Input: part model. Units: mm. Frame: model coordinates. A direction names the side the tool comes from. Coordinates: 2 decimals unless noted, no trailing zeros. Loops run counter-clockwise (first coordinate to the right, second up) from the corner with the lowest first, then second, coordinate; pieces in that order, holes last. Notation, with made-up numbers: (5, 8) - (39, 8) arc R13 ccw to (39, 31) - close; hole circle Ø3 at (-16.5, 26). An arc over 180 degrees is marked (long way). Answer as CSV lines item,"result". Start each with the question number.
```python
from build123d import *

# Parameters (mm, degrees)
F1_DEPTH  = 3.5
F2_W      = 29
F2_H      = 9
F3_DEPTH  = 4
F4_W      = 29
F4_H      = 9
F5_DEPTH  = 4
F6_SIZE   = 2
F7_W      = 4
F7_H      = 15
F8_DEPTH  = 3
F9_SIZE   = 2
F11_DEPTH = 29
F12_R     = 3


with BuildPart() as f1:
    # F0 (on Top) → F1 (new body)
    with BuildSketch(Plane.XY):
        Polygon((-4.25, 12.1511180716), (-18, 12.1511180716), (-18, -16.8488819284), (-11.125, -16.8488819284), (-11.125, -12.8488819284), (11.125, -12.8488819284), (11.125, -16.8488819284), (18, -16.8488819284), (18, 12.1511180716), (4.25, 12.1511180716), (4.25, 7.1511180716), (-4.25, 7.1511180716), align=None)
    extrude(amount=F1_DEPTH)

    # F2 (on face) → F3 (join)
    with BuildSketch(Plane(origin=(-18, 0, 0), x_dir=(0, -1, 0), z_dir=(-1, 0, 0))):
        with Locations((2.3488819284, -1)):
            Rectangle(F2_W, F2_H)
    extrude(amount=F3_DEPTH)

    # F4 (on face) → F5 (join)
    with BuildSketch(Plane.YZ.offset(18)):
        with Locations((-2.3488819284, -1)):
            Rectangle(F4_W, F4_H)
    extrude(amount=F5_DEPTH)

    # F6
    f6_edges = [f1.edges().sort_by_distance(p)[0] for p in [
        (-14.5625, -16.848882, 0),
        (14.5625, -16.848882, 0),
    ]]
    chamfer(f6_edges, length=F6_SIZE)

    # F7 (on face) → F8 (join)
    with BuildSketch(Plane(origin=(0, 0, -5.5), x_dir=(1, 0, 0), z_dir=(0, 0, -1))):
        with Locations((20, 2.3488819284)):
            Rectangle(F7_W, F7_H)
        with Locations((-20, 2.3488819284)):
            Rectangle(F7_W, F7_H)
    extrude(amount=F8_DEPTH)

    # F9
    f9_edges = [f1.edges().sort_by_distance(p)[0] for p in [
        (18, -16.848882, -1.75),
        (-18, -16.848882, -1.75),
    ]]
    chamfer(f9_edges, length=F9_SIZE)

    # F10 (on face) → F11 (join, through all)
    with BuildSketch(Plane(origin=(0, 12.1511180716, 0), x_dir=(-1, 0, 0), z_dir=(0, 1, 0))):
        Polygon((25, -5.5), (22, 3.5), (22, -5.5), align=None)
        Polygon((-22, -5.5), (-22, 3.5), (-25, -5.5), align=None)
    extrude(amount=-F11_DEPTH)

    # F12
    f12_edges = [f1.edges().sort_by_distance(p)[0] for p in [
        (-22, -2.348882, 3.5),
        (22, -2.348882, 3.5),
    ]]
    fillet(f12_edges, radius=F12_R)


solid = f1.part
```
Item 1: Section query D-D, the plane x = 16. Output: boundary loops of the cut face in (y, z), and give its area (3 significant figures).
Item 2: Set-up query: faces 4 (the flat face through (-20, 5.151, -7)), 5 (the flat face through (-11.125, -14, 2)), 6 (the flat face through (-22, -2, -7)), 7 (the flat face through (20, -9.849, -7)), 8 (the flat face through (-18.986, -15.835, -2.636)). Return all of +Z, -Z, +X, -X, +Y, -Y with unobstructed straight access to the full face (end or side cutting, diameter ignored); none if empty.
Item 3: Contact query for flat-ended pins moving along their axis: P1, Ø0.9, axis at y = -6, z = -6.5, coming from the -X side; P2, Ø1.5, axis at y = -4, z = 1.5, coming from the +X side; P3, Ø2, axis at y = 5.5, z = -2, coming from the +X side; P4, Ø2.5, axis at y = -5, z = -6.5, coming from the +X side. Output: stop coordinate, or through.
Item 4: Section query A-A, the plane z = -1. Output: boundary loops of the cut face in (x, y).
Item 5: Section query C-C, the plane y = -12.25. Output: boundary loops of the cut face in (x, z).
Item 6: Section query B-B, the plane y = 8. Output: boundary loops of the cut face in (x, z).
Item 7: Draft query along X for faces 1 (the cylindrical face through (-21.61, -2.55, 2.92)), 2 (the flat face through (20, -2, -8.5)), 3 (the flat face through (0, -1, 0)). Return one class per face: pulls with the +X half, pulls with the -X half, needs draft (parallel to the pull), parting line crosses it, or undercut.
Item 8: Material intervals for probe 1 along Z at (x, y) = (15, -7); probe 2 along X at (y, z) = (-8.75, -5.75); probe 3 along X at (y, z) = (8.5, 1.5), sorted ascending.
Response values:
1,outline,"(-16.85, 2) - (-14.85, 0) - (12.15, 0) - (12.15, 3.5) - (-16.85, 3.5) - close"
1,area,"99.5 mm²"
2,face 4,"-Z, +X, -X, +Y"
2,face 5,"+Z, -Z, -Y"
2,face 6,"-Z, -X, +Y, -Y"
2,face 7,"-Z, +X, -X, -Y"
2,face 8,"-Z, -Y"
3,P1,"stops at x = -22"
3,P2,"stops at x = 22.92"
3,P3,"stops at x = 24.17"
3,P4,"stops at x = 25"
4,outline,"(-23.5, -16.85) - (-20, -16.85) - (-18, -14.85) - (-18, 12.15) - (-23.5, 12.15) - close; (18, -14.85) - (20, -16.85) - (23.5, -16.85) - (23.5, 12.15) - (18, 12.15) - close"
5,outline,"(-25, -5.5) - (-18, -5.5) - (-18, 0) - (18, 0) - (18, -5.5) - (25, -5.5) - (22.68, 1.45) arc R3 ccw to (19.84, 3.5) - (-19.84, 3.5) arc R3 ccw to (-22.68, 1.45) - close"
6,outline,"(-25, -5.5) - (-18, -5.5) - (-18, 0) - (-4.25, 0) - (-4.25, 3.5) - (-19.84, 3.5) arc R3 ccw to (-22.68, 1.45) - close; (4.25, 0) - (18, 0) - (18, -5.5) - (25, -5.5) - (22.68, 1.45) arc R3 ccw to (19.84, 3.5) - (4.25, 3.5) - close"
7,face 1,"pulls with the -X half"
7,face 2,"needs draft"
7,face 3,"undercut"
8,probe 1,"z = 0 to 3.5"
8,probe 2,"x = -22 to -18, 18 to 22"
8,probe 3,"x = -22.67 to -4.25, 4.25 to 22.67"
